Read the model definition and answer for the solid it produces. Units are mm, in the model's axes. Give positions to 0.01 mm unless a question says otherwise; leave off trailing zeros. Write each loop counter-clockwise with the first axis right and the second up, starting at its lowest first coordinate (ties: lowest second). Pieces come first, ordered by that corner, then holes.
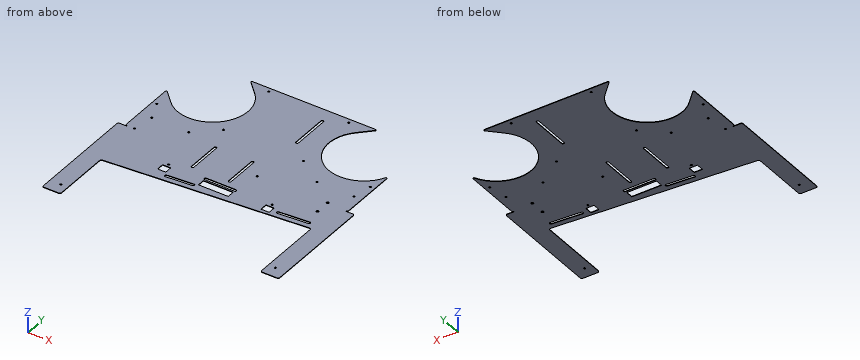
```python
from build123d import *

# Parameters (mm, degrees)
MODEL_R            = 1.25
MODEL_R_2          = 1.7
BASE_FLANGE1_DEPTH = 0.635


# Sheet-metal steps are written as plain solids
with BuildPart() as part:
    # Model → Base-Flange1 (new body)
    with BuildSketch(Plane.XY):
        with BuildLine():
            Line((0, 130.410642225), (0, 52.635))
            ThreePointArc((0, 52.635), (0.585786438, 51.220786438), (2, 50.635))
            Line((2, 50.635), (2.6416, 50.635))
            Line((2.6416, 50.635), (2.6416, 50))
            Line((2.6416, 50), (-7.411304242, 50))
            ThreePointArc((-7.411304242, 50), (-8.825517804, 49.414213562), (-9.411304242, 48))
            Line((-9.411304242, 48), (-9.411304242, -98))
            ThreePointArc((-9.411304242, -98), (-8.825517804, -99.414213562), (-7.411304242, -100))
            Line((-7.411304242, -100), (12.92885, -100))
            ThreePointArc((12.92885, -100), (14.343063562, -99.414213562), (14.92885, -98))
            Line((14.92885, -98), (14.92885, -21.852062278))
            ThreePointArc((14.92885, -21.852062278), (15.461405624, -20.493163091), (16.775457002, -19.857953307))
            Line((16.775457002, -19.857953307), (281.917757002, 0.537608254))
            ThreePointArc((281.917757002, 0.537608254), (283.430049188, 0.01094366), (284.07115, -1.456500717))
            Line((284.07115, -1.456500717), (284.07115, -98))
            ThreePointArc((284.07115, -98), (284.656936438, -99.414213562), (286.07115, -100))
            Line((286.07115, -100), (306.411304242, -100))
            ThreePointArc((306.411304242, -100), (307.825517804, -99.414213562), (308.411304242, -98))
            Line((308.411304242, -98), (308.411304242, 48))
            ThreePointArc((308.411304242, 48), (307.825517804, 49.414213562), (306.411304242, 50))
            Line((306.411304242, 50), (296.3584, 50))
            Line((296.3584, 50), (296.3584, 50.635))
            Line((296.3584, 50.635), (297, 50.635))
            ThreePointArc((297, 50.635), (298.414213562, 51.220786438), (299, 52.635))
            Line((299, 52.635), (299, 128.371893989))
            ThreePointArc((299, 128.371893989), (298.220121803, 129.347366383), (297.096907217, 128.801339474))
            ThreePointArc((297.096907217, 128.801339474), (226.808500251, 110.393354416), (220.612427894, 182.787572106))
            Line((220.612427894, 182.787572106), (236.117749006, 198.292893219))
            ThreePointArc((236.117749006, 198.292893219), (236.334521757, 199.382683432), (235.410642225, 200))
            Line((235.410642225, 200), (69.589357776, 200))
            ThreePointArc((69.589357776, 200), (68.665478243, 199.382683432), (68.882250994, 198.292893219))
            Line((68.882250994, 198.292893219), (84.387572107, 182.787572107))
            ThreePointArc((84.387572107, 182.787572107), (84.387572107, 115.612427894), (17.212427894, 115.612427894))
            Line((17.212427894, 115.612427894), (1.707106781, 131.117749006))
            ThreePointArc((1.707106781, 131.117749006), (0.617316568, 131.334521758), (0, 130.410642225))
        make_face()
        with Locations((177.3, 51)):
            Circle(MODEL_R, mode=Mode.SUBTRACT)
        with Locations((12.3, 51)):
            Circle(MODEL_R, mode=Mode.SUBTRACT)
        with Locations((271, 32.2)):
            Circle(MODEL_R_2, mode=Mode.SUBTRACT)
        with Locations((271, 52.2)):
            Circle(MODEL_R_2, mode=Mode.SUBTRACT)
        with Locations((5.25, -84.9)):
            Circle(MODEL_R, mode=Mode.SUBTRACT)
        with Locations((293.75, -84.9)):
            Circle(MODEL_R, mode=Mode.SUBTRACT)
        with Locations((83, 14.351626942)):
            Circle(MODEL_R, mode=Mode.SUBTRACT)
        with Locations((222, 14.351626942)):
            Circle(MODEL_R, mode=Mode.SUBTRACT)
        with Locations((238.6616, 78.8319)):
            Circle(MODEL_R, mode=Mode.SUBTRACT)
        with Locations((16.3384, 78.8315)):
            Circle(MODEL_R, mode=Mode.SUBTRACT)
        with Locations((203.3563, 104.3563)):
            Circle(MODEL_R, mode=Mode.SUBTRACT)
        with Locations((95.6437, 104.3563)):
            Circle(MODEL_R, mode=Mode.SUBTRACT)
        with Locations((95.6437, 194.0437)):
            Circle(MODEL_R, mode=Mode.SUBTRACT)
        with Locations((5.9563, 104.3563)):
            Circle(MODEL_R, mode=Mode.SUBTRACT)
        with Locations((203.3563, 194.0437)):
            Circle(MODEL_R, mode=Mode.SUBTRACT)
        with Locations((293.0437, 104.3563)):
            Circle(MODEL_R, mode=Mode.SUBTRACT)
        with Locations((66.3384, 78.8315)):
            Circle(MODEL_R, mode=Mode.SUBTRACT)
        with Locations((288.6616, 78.8319)):
            Circle(MODEL_R, mode=Mode.SUBTRACT)
        with BuildLine():
            Line((179, 130), (179, 180))
            ThreePointArc((179, 180), (177.3, 181.7), (175.6, 180))
            Line((175.6, 180), (175.6, 130))
            ThreePointArc((175.6, 130), (177.3, 128.3), (179, 130))
        make_face(mode=Mode.SUBTRACT)
        with BuildLine():
            Line((155.85, 70.582396166), (155.85, 25.582396166))
            ThreePointArc((155.85, 25.582396166), (157.5, 23.932396166), (159.15, 25.582396166))
            Line((159.15, 25.582396166), (159.15, 70.582396166))
            ThreePointArc((159.15, 70.582396166), (157.5, 72.232396166), (155.85, 70.582396166))
        make_face(mode=Mode.SUBTRACT)
        with BuildLine():
            Line((109.15, 25.582396166), (109.15, 70.582396166))
            ThreePointArc((109.15, 70.582396166), (107.5, 72.232396166), (105.85, 70.582396166))
            Line((105.85, 70.582396166), (105.85, 25.582396166))
            ThreePointArc((105.85, 25.582396166), (107.5, 23.932396166), (109.15, 25.582396166))
        make_face(mode=Mode.SUBTRACT)
        with BuildLine():
            Line((172.5, 16.051626942), (132.5, 16.051626942))
            ThreePointArc((132.5, 16.051626942), (130.8, 14.351626942), (132.5, 12.651626942))
            Line((132.5, 12.651626942), (172.5, 12.651626942))
            ThreePointArc((172.5, 12.651626942), (174.2, 14.351626942), (172.5, 16.051626942))
        make_face(mode=Mode.SUBTRACT)
        with BuildLine():
            Line((275.699508159, 10.287481051), (235.81732874, 7.219621092))
            ThreePointArc((235.81732874, 7.219621092), (234.252720163, 5.394244419), (236.078096836, 3.829635842))
            Line((236.078096836, 3.829635842), (275.960276256, 6.8974958))
            ThreePointArc((275.960276256, 6.8974958), (277.524884833, 8.722872474), (275.699508159, 10.287481051))
        make_face(mode=Mode.SUBTRACT)
        with BuildLine():
            Line((77.5, 0.851626942), (77.5, 9.851626942))
            ThreePointArc((77.5, 9.851626942), (77.64644661, 10.205180332), (78, 10.351626942))
            Line((78, 10.351626942), (88, 10.351626942))
            ThreePointArc((88, 10.351626942), (88.353553391, 10.205180332), (88.5, 9.851626942))
            Line((88.5, 9.851626942), (88.5, 0.851626942))
            ThreePointArc((88.5, 0.851626942), (88.353553391, 0.498073551), (88, 0.351626942))
            Line((88, 0.351626942), (78, 0.351626942))
            ThreePointArc((78, 0.351626942), (77.64644661, 0.498073551), (77.5, 0.851626942))
        make_face(mode=Mode.SUBTRACT)
        with BuildLine():
            Line((216.5, 9.851626942), (216.5, 0.851626942))
            ThreePointArc((216.5, 0.851626942), (216.64644661, 0.498073551), (217, 0.351626942))
            Line((217, 0.351626942), (227, 0.351626942))
            ThreePointArc((227, 0.351626942), (227.353553391, 0.498073551), (227.5, 0.851626942))
            Line((227.5, 0.851626942), (227.5, 9.851626942))
            ThreePointArc((227.5, 9.851626942), (227.353553391, 10.205180332), (227, 10.351626942))
            Line((227, 10.351626942), (217, 10.351626942))
            ThreePointArc((217, 10.351626942), (216.64644661, 10.205180332), (216.5, 9.851626942))
        make_face(mode=Mode.SUBTRACT)
        with BuildLine():
            Line((132.5, 9.851626942), (132.5, 0.851626942))
            ThreePointArc((132.5, 0.851626942), (132.64644661, 0.498073551), (133, 0.351626942))
            Line((133, 0.351626942), (172, 0.351626942))
            ThreePointArc((172, 0.351626942), (172.353553391, 0.498073551), (172.5, 0.851626942))
            Line((172.5, 0.851626942), (172.5, 9.851626942))
            ThreePointArc((172.5, 9.851626942), (172.353553391, 10.205180332), (172, 10.351626942))
            Line((172, 10.351626942), (133, 10.351626942))
            ThreePointArc((133, 10.351626942), (132.64644661, 10.205180332), (132.5, 9.851626942))
        make_face(mode=Mode.SUBTRACT)
        with BuildLine():
            Line((127.875303432, -4.493655968), (92.97839644, -7.178033432))
            ThreePointArc((92.97839644, -7.178033432), (91.153019766, -5.613424855), (92.717628343, -3.788048182))
            Line((92.717628343, -3.788048182), (127.614535335, -1.103670718))
            ThreePointArc((127.614535335, -1.103670718), (129.439912009, -2.668279295), (127.875303432, -4.493655968))
        make_face(mode=Mode.SUBTRACT)
    extrude(amount=-BASE_FLANGE1_DEPTH)


solid = part.part
```
Item 1: This flat-tipped pin is pushed along its axis until it touches: pin 1 Ø1.5 at (x, y) = (288.66, 78.83) entering from -Z. Where does it stop, or does it pass through?
Result set:
pin 1: passes through
Item 2: Section B-B (y = -49) is taken. Write down the section's boundary in (x, z) (3 decimals), and give its area (3 significant figures).
Result set:
outline: (-9.411, -0.635) - (14.929, -0.635) - (14.929, 0) - (-9.411, 0) - close; (284.071, -0.635) - (308.411, -0.635) - (308.411, 0) - (284.071, 0) - close
area: 30.9 mm2
Item 3: Section C-C (x = 254.2) is taken. Write down the section's boundary in (y, z) (3 decimals).
Result set:
outline: (-1.595, -0.635) - (5.224, -0.635) - (5.224, 0) - (-1.595, 0) - close; (8.634, -0.635) - (101.7, -0.635) - (101.7, 0) - (8.634, 0) - close
Item 4: Section A-A (y = 65) is taken. Write down the section's boundary in (x, z) (3 decimals), and give its area (3 significant figures).
Result set:
outline: (0, -0.635) - (105.85, -0.635) - (105.85, 0) - (0, 0) - close; (109.15, -0.635) - (155.85, -0.635) - (155.85, 0) - (109.15, 0) - close; (159.15, -0.635) - (299, -0.635) - (299, 0) - (159.15, 0) - close
area: 186 mm2
Item 5: Section D-D (z = -0.35) is taken. Give the number of separate pieces and of enclosed holes in the cut face, and give its area (3 significant figures).
Result set:
separate pieces: 1
enclosed holes: 27
area: 50,800 mm2
Item 6: Find the intervals of material crossed by line 1 along X through (y, z) = (51.5, -0.1); line 2 along Y through (x, z) = (219.5, -0.05); line 3 along Y through (x, z) = (177.3, -0.2), in increasing order.
Result set:
line 1: x = 0.35 to 11.15, 13.45 to 105.85, 109.15 to 155.85, 159.15 to 176.15, 178.45 to 269.45, 272.55 to 298.65
line 2: y = -4.26 to 0.35, 10.35 to 116.76, 181.64 to 200
line 3: y = -7.51 to 49.75, 52.25 to 128.3, 181.7 to 200
